The drawing under review shows one solid part. Ordinate dimensions are in mm from its lowest x, y, z. A direction names the side the tool comes from. Give positions to 0.01 mm unless a question says otherwise; leave off trailing zeros. Write each loop counter-clockwise with the first axis right and the second up, starting at its lowest first coordinate (ties: lowest second). Pieces come first, ordered by that corner, then holes. Notation, with made-up numbers: (83.25, 73.25) - (98.25, 73.25) arc R21 cw to (98.25, 112.25) - close; hole circle Ø2 at (9.5, 46.5). An arc over 180 degrees is marked (long way). Write item = value, one per line.
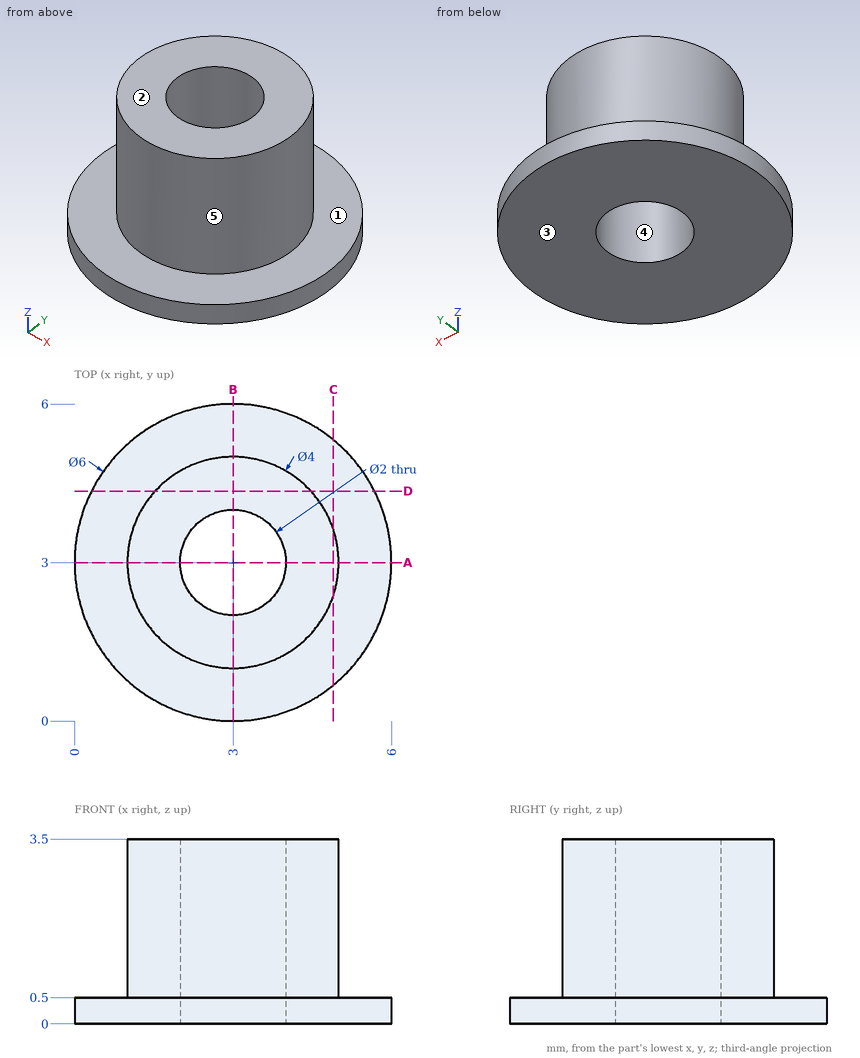
1. For line 1 (Y direction, x = 3, z = 2.45); line 2 (Z direction, x = 4.5, y = 1.5); line 3 (X direction, y = 3.6, z = 2.1), list the stretches that pass through material, from the lowest coordinate up. Write a range as from..to.
Findings below:
line_1 = 1..2, 4..5
line_2 = 0..0.5
line_3 = 1.09..2.2, 3.8..4.91
2. Take a section at A-A on y = 3. Give the boundary of the cut face in (x, z), and give its area (3 significant figures).
Findings below:
outline = (0, 0) - (2, 0) - (2, 3.5) - (1, 3.5) - (1, 0.5) - (0, 0.5) - close; (4, 0) - (6, 0) - (6, 0.5) - (5, 0.5) - (5, 3.5) - (4, 3.5) - close
area = 8.00 mm²
3. Insertion check: P1, Ø1, axis at x = 3, z = 1.5, coming from the +Y side; P2, Ø1.5, axis at y = 1, z = 1.5, coming from the +X side. Each pin has a flat end and moves straight along its axis. Give the tip position at first contact, or say it passes through.
Findings below:
P1 = 5
P2 = 4.56
4. Draft analysis for pull direction Y (two halves, no side actions). For the marked faces 3, 4 and 5, state which applies: +Y half, -Y half, draft (parallel to the pull), parting line (faces both ways), or undercut.
Findings below:
face_3 = draft
face_4 = undercut
face_5 = parting line
5. Take a section at D-D on y = 4.35. Give the boundary of the cut face in (x, z).
Findings below:
outline = (0.32, 0) - (5.68, 0) - (5.68, 0.5) - (4.48, 0.5) - (4.48, 3.5) - (1.52, 3.5) - (1.52, 0.5) - (0.32, 0.5) - close
6. Take a section at C-C on x = 4.9. Give the boundary of the cut face in (y, z).
Findings below:
outline = (0.68, 0) - (5.32, 0) - (5.32, 0.5) - (3.62, 0.5) - (3.62, 3.5) - (2.38, 3.5) - (2.38, 0.5) - (0.68, 0.5) - close
7. Machinability: for the marked faces 1 and 2, which of the approach directions +Z, -Z, +X, -X, +Y, -Y give a long, thin tool a straight path to every point of the face, cutting with its end or side? Answer none if there is none.
Findings below:
face_1 = +Z
face_2 = +Z, +X, -X, +Y, -Y
